The model under review builds one solid part; all positions refer to its coordinate system, in mm. A direction names the side the tool comes from. Round coordinates to 2 decimals unless told otherwise and drop trailing zeros. Order: outer loops, then holes, each group sorted by start corner. A loop starts at its lowest first (then second) coordinate and runs counter-clockwise, first axis right, second up. Notation, with made-up numbers: M 49,26 L 54,26 A23 ccw 54,65 Z; hole C -30.75,-31 d8. An arc over 180 degrees is marked long. Answer as a JSON object with one key per item and string values. Group by question number.
1. Add section D-D on x = 1.5. State the section outline as (y, z) points, and give its area (3 significant figures).
2. Add section A-A on y = 0. State the section outline as (x, z) points (3 decimals).
3. Clearance check with a flat-ended pin moving along its axis: P1, Ø0.6, axis at x = 0.5, z = 1.5, coming from the +Y side. State where the tip first meets the part, or that it passes through.
4. Add section B-B on x = -0.9. State the section outline as (y, z) points, and give its area (3 significant figures).
5. Machinability: for faces 1 (the face through (0.65, 1.01, 2.25)), 2 (the face through (0, 0, 0)), which of the approach directions +Z, -Z, +X, -X, +Y, -Y give a long, thin tool a straight path to every point of the face, cutting with its end or side? Answer none if there is none.
6. Add section C-C on z = 2.3. State the section outline as (x, y) points, and give its area (3 significant figures).
7. To check wall thickness, follow probe 1 along Z at (x, y) = (-1.2, 1); probe 2 along Y at (x, z) = (-1.35, 1.9); probe 3 along Y at (x, z) = (0.4, 0.3). State the ranges of each line that lie inside material, in increasing order. Write a range as [from, to].
```python
from build123d import *

# Parameters (mm, degrees)
F0_W          = 3.81
F0_H          = 6.2
F1_DEPTH      = 2
F2_R          = 1.2
F3_DEPTH      = 0.5
F5_DEPTH      = 0.6
F5_DEPTH_BACK = 0.6


with BuildPart() as f1:
    # F0 (on Top) → F1 (new body)
    with BuildSketch(Plane.XY):
        Rectangle(F0_W, F0_H)
    extrude(amount=F1_DEPTH)

    # F2 (on face) → F3 (join)
    with BuildSketch(Plane.XY.offset(2)):
        Circle(F2_R)
    extrude(amount=F3_DEPTH)

    # F4 (on Right) → F5 (join, two sides)
    with BuildSketch(Plane.YZ) as f5_sk:
        with BuildLine():
            Line((3.384861, 0.4), (3.1, 0.4))
            Line((3.1, 0.4), (3.1, 0.2))
            Line((3.1, 0.2), (3.384861, 0.2))
            ThreePointArc((3.384861, 0.2), (3.39935, 0.197855), (3.412596, 0.191603))
            Line((3.412596, 0.191603), (3.687404, 0.008397))
            ThreePointArc((3.687404, 0.008397), (3.70065, 0.002145), (3.715139, 0))
            Line((3.715139, 0), (3.95, 0))
            ThreePointArc((3.95, 0), (3.985355, 0.014645), (4, 0.05))
            Line((4, 0.05), (4, 0.15))
            ThreePointArc((4, 0.15), (3.985355, 0.185355), (3.95, 0.2))
            Line((3.95, 0.2), (3.715139, 0.2))
            ThreePointArc((3.715139, 0.2), (3.70065, 0.202145), (3.687404, 0.208397))
            Line((3.687404, 0.208397), (3.412596, 0.391603))
            ThreePointArc((3.412596, 0.391603), (3.39935, 0.397855), (3.384861, 0.4))
        make_face()
    extrude(amount=F5_DEPTH)
    extrude(f5_sk.sketch, amount=-F5_DEPTH_BACK)

    # F6: F1 across plane


with BuildPart() as f1_1:
    add(f1.part)
    add(f1.part.mirror(Plane.XZ))


solid = f1_1.part
```
Recorded:
{
 "1": {"outline": "M -3.1,0 L 3.1,0 L 3.1,2 L -3.1,2 Z", "area": "12.4 mm²"},
 "2": {"outline": "M -1.905,0 L 1.905,0 L 1.905,2 L 1.2,2 L 1.2,2.5 L -1.2,2.5 L -1.2,2 L -1.905,2 Z"},
 "3": {"P1": "stops at y = 3.1"},
 "4": {"outline": "M -3.1,0 L 3.1,0 L 3.1,2 L 0.79,2 L 0.79,2.5 L -0.79,2.5 L -0.79,2 L -3.1,2 Z", "area": "13.2 mm²"},
 "5": {"face 1": "+Z", "face 2": "-Z, +X, -X, +Y, -Y"},
 "6": {"outline": "C 0,0 d2.4", "area": "4.52 mm²"},
 "7": {"probe 1": "z = [0, 2]", "probe 2": "y = [-3.1, 3.1]", "probe 3": "y = [-3.55, 3.55]"}
}
